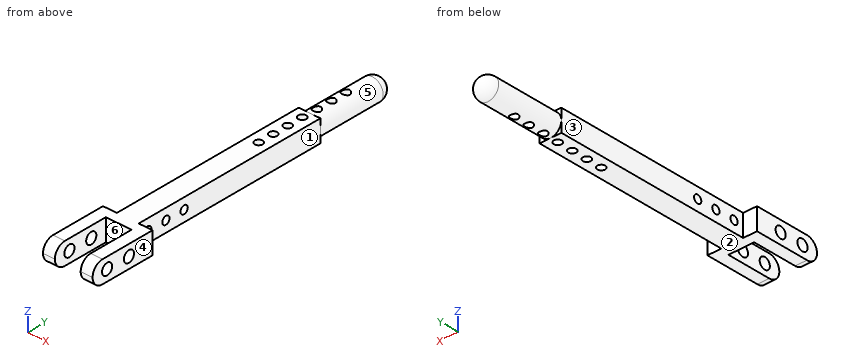
```python
from build123d import *

# Parameters (mm, degrees)
BOSS_EXTRUDE1_DEPTH = 5.5
SKETCH2_R           = 1
CUT_EXTRUDE1_DEPTH  = 5.5
SKETCH3_R           = 1.4
CUT_EXTRUDE2_DEPTH  = 20
SKETCH4_R           = 2.75
BOSS_EXTRUDE2_DEPTH = 20
FILLET1_R           = 2.75
FILLET2_R           = 2.75
SKETCH6_R           = 1
CUT_EXTRUDE4_DEPTH  = 10


with BuildPart() as part:
    # Sketch1 → Boss-Extrude1 (new body)
    with BuildSketch(Plane.XY):
        Polygon((-6.25, -1.20199904), (-6.25, -17.70199904), (-3.25, -17.70199904), (-3.25, -3.70199904), (3.25, -3.70199904), (3.25, -17.70199904), (6.25, -17.70199904), (6.25, -1.20199904), (2.75, -1.20199904), (2.75, 48.79800096), (-2.75, 48.79800096), (-2.75, -1.20199904), align=None)
    extrude(amount=BOSS_EXTRUDE1_DEPTH)

    # Sketch2 → Cut-Extrude1 (cut)
    with BuildSketch(Plane(origin=(2.75, 0, 0), x_dir=(0, 0, -1), z_dir=(1, 0, 0))):
        with Locations((-2.75, 1.29800096)):
            Circle(SKETCH2_R)
        with Locations((-2.75, 6.29800096)):
            Circle(SKETCH2_R)
        with Locations((-2.75, 11.29800096)):
            Circle(SKETCH2_R)
    extrude(amount=-CUT_EXTRUDE1_DEPTH, mode=Mode.SUBTRACT)

    # Sketch3 → Cut-Extrude2 (cut)
    with BuildSketch(Plane(origin=(6.25, 0, 0), x_dir=(0, 0, -1), z_dir=(1, 0, 0))):
        with Locations(Location((-2.75, -7.70199904, 0), (0, 0, 90))):
            Circle(SKETCH3_R)
        with Locations(Location((-2.75, -13.70199904, 0), (0, 0, 90))):
            Circle(SKETCH3_R)
    extrude(amount=-CUT_EXTRUDE2_DEPTH, mode=Mode.SUBTRACT)

    # Sketch4 → Boss-Extrude2 (add)
    with BuildSketch(Plane(origin=(0, 48.79800096, 0), x_dir=(1, 0, 0), z_dir=(0, 1, 0))):
        with Locations(Location((0, -2.75, 0), (0, 0, 270))):
            Circle(SKETCH4_R)
    extrude(amount=BOSS_EXTRUDE2_DEPTH)

    # Fillet1
    fillet1_edges = [part.edges().sort_by_distance(p)[0] for p in [
        (0, 68.79800096, 0),
    ]]
    fillet(fillet1_edges, radius=FILLET1_R)

    # Fillet2
    fillet2_edges = [part.edges().sort_by_distance(p)[0] for p in [
        (4.75, -17.70199904, 5.5),
        (4.75, -17.70199904, 0),
        (-4.75, -17.70199904, 0),
        (-4.75, -17.70199904, 5.5),
    ]]
    fillet(fillet2_edges, radius=FILLET2_R - 0.0001)  # a hair under: the kernel refuses the full size

    # Sketch6 → Cut-Extrude4 (cut)
    with BuildSketch(Plane(origin=(0, 0, 0), x_dir=(-1, 0, 0), z_dir=(0, 0, -1))):
        with Locations((0, 46.79800096)):
            Circle(SKETCH6_R)
        with Locations((0, 42.79800096)):
            Circle(SKETCH6_R)
        with Locations((0, 38.79800096)):
            Circle(SKETCH6_R)
        with Locations((0, 34.79800096)):
            Circle(SKETCH6_R)
        with Locations((0, 50.79800096)):
            Circle(SKETCH6_R)
        with Locations((0, 54.79800096)):
            Circle(SKETCH6_R)
        with Locations((0, 58.79800096)):
            Circle(SKETCH6_R)
    extrude(amount=-CUT_EXTRUDE4_DEPTH, mode=Mode.SUBTRACT)


solid = part.part
```
Could you check a few things on this model? Use its own coordinates, in mm. Face numbers are marked on the shaded views. A direction names the side the tool comes from. Coordinates: 2 decimals unless noted, no trailing zeros. Order: outer loops, then holes, each group sorted by start corner. A loop starts at its lowest first (then second) coordinate and runs counter-clockwise, first axis right, second up. Notation, with made-up numbers: M 1.5,-18 L 29.5,-18 A14 ccw 29.5,0 Z; hole C 50.25,77.5 d7. An arc over 180 degrees is marked long. Use a Markdown table: item, result. Add a question column.
Q1. I'm going to push flat-ended pins straight in: pin 1 (2 mm diameter, centred on x = 2, z = 3, fed in from +Y); pin 2 (3 mm diameter, centred on y = 1.298, z = 2.75, fed in from -X); pin 3 (6 mm diameter, centred on x = 5, y = 33, fed in from -Z); pin 4 (3 mm diameter, centred on y = 59.5, z = 1.5, fed in from -X). Where does each tip first touch, or does it pass through?
Q2. We'd pull the mould along X, two halves only. Please class the marked faces 4, 5 and 6: pulls with the +X half, pulls with the -X half, needs draft (parallel to the pull), parting line crosses it, or undercut.
Q3. I want a section at B-B on y = 33. List the corners of the cut face in (x, z) for me.
Q4. Which directions (+Z, -Z, +X, -X, +Y, -Y) give clear straight access to the entire face, cutting with the end or side of a thin tool? Please do the marked faces 1, 2 and 3.
Q5. I want a section at A-A on x = 4.5. Give the number of separate pieces and of enclosed holes in the cut face, then the cut area to 3 significant figures.
Q6. If I drill on L1, parallel to X at y = -6, z = 0.7; L2, parallel to Y at x = 1.25, z = 1.9; L3, parallel to X at y = 44, z = 2.55, over which ranges is the centre line in solid material (lowest first)?
Checked values:
| question | item | result |
|---|---|---|
| 1 | pin 1 | y = 68.6 |
| 1 | pin 2 | x = -2.75 |
| 1 | pin 3 | z = 0 |
| 1 | pin 4 | x = -2.75 |
| 2 | face 4 | pulls with the +X half |
| 2 | face 5 | parting line crosses it |
| 2 | face 6 | undercut |
| 3 | outline | M -2.75,0 L 2.75,0 L 2.75,5.5 L -2.75,5.5 Z |
| 4 | face 1 | +Z, -Z, +X, +Y |
| 4 | face 2 | -Z, +X, -X, +Y, -Y |
| 4 | face 3 | +Z, -Z, -X, +Y |
| 5 | separate pieces | 1 |
| 5 | enclosed holes | 2 |
| 5 | area | 75.2 mm² |
| 6 | L1 | -6.25 to -3.25, 3.25 to 6.25 |
| 6 | L2 | -3.7 to 0.77, 1.82 to 5.77, 6.82 to 10.77, 11.82 to 68.35 |
| 6 | L3 | -2.75 to 2.75 |
